Can you work these out from the drawing? Everything is in mm from the part's minimum corner. A direction names the side the tool comes from. Coordinates: 2 decimals unless noted, no trailing zeros. Loops run counter-clockwise (first coordinate to the right, second up) from the corner with the lowest first, then second, coordinate; pieces in that order, holes last.
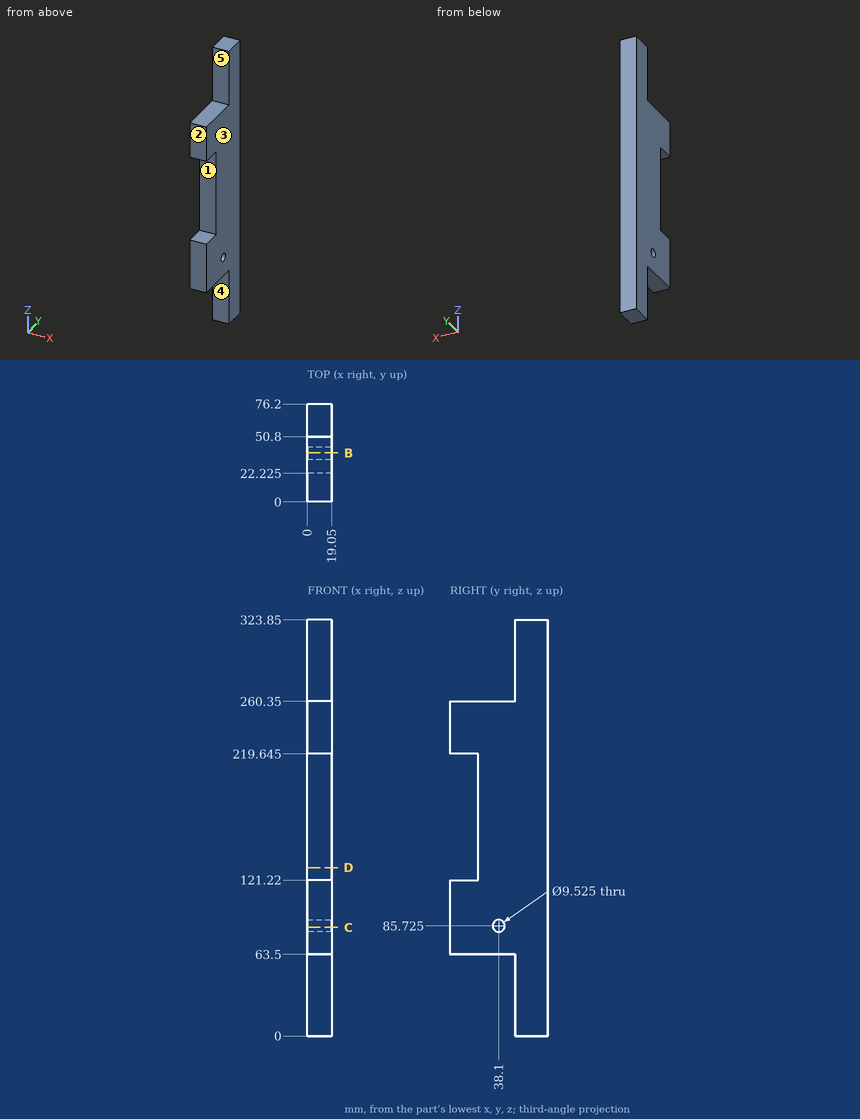
1. I want a section at C-C (z = 84.5). Please give me the cut outline in (x, y), then the cut area to 3 significant figures.
2. We'd pull the mould along Z, two halves only. Please class the marked faces 1 and 2: +Z half, -Z half, draft (parallel to the pull), parting line (faces both ways), or undercut.
3. For pin 1 (1 mm diameter, centred on x = 10.5, y = 29, fed in from +Z); pin 2 (6 mm diameter, centred on x = 13.5, y = 11, fed in from -Z); pin 3 (9.5 mm diameter, centred on x = 6, z = 282.5, fed in from -Y), each with a flat end and sliding along its axis, tell me the tip position at first contact or that it passes through.
4. On a 3-axis mill with a long thin cutter (end or side, diameter ignored), from which of +Z, -Z, +X, -X, +Y, -Y can I reach the whole of each face in a straight line? I mean the marked faces 3, 4 and 5. Say none if no direction works.
5. I want a section at B-B (y = 38.1). Please give me the cut outline in (x, z), then the cut area to 3 significant figures.
6. I need wall thicknesses on line 1 along Y through (x, z) = (4.25, 48); line 2 along Y through (x, z) = (3.25, 180.5) (3 decimals); line 3 along Y through (x, z) = (8.25, 82). Which ranges of each line are inside material? Lowest first, please.
7. I want a section at D-D (z = 131). Please give me the cut outline in (x, y) (3 decimals).
Response values:
1. outline: (0, 0) - (19.05, 0) - (19.05, 33.5) - (0, 33.5) - close; (0, 42.7) - (19.05, 42.7) - (19.05, 76.2) - (0, 76.2) - close
1. area: 1,280 mm2
2. face 1: undercut
2. face 2: draft
3. pin 1: stops at z = 260.35
3. pin 2: stops at z = 63.5
3. pin 3: stops at y = 50.8
4. face 3: +Z, -Z, +X, +Y, -Y
4. face 4: -Z, +X, -X, -Y
4. face 5: +Z, +X, -X, -Y
5. outline: (0, 63.5) - (19.05, 63.5) - (19.05, 80.96) - (0, 80.96) - close; (0, 90.49) - (19.05, 90.49) - (19.05, 260.35) - (0, 260.35) - close
5. area: 3,570 mm2
6. line 1: y = 50.8 to 76.2
6. line 2: y = 22.225 to 76.2
6. line 3: y = 0 to 35.13, 41.07 to 76.2
7. outline: (0, 22.225) - (19.05, 22.225) - (19.05, 76.2) - (0, 76.2) - close
